Could you check a few things on this model? Use its own coordinates, in mm. Face numbers are marked on the shaded views. Round coordinates to 2 decimals unless told otherwise and drop trailing zeros. Order: outer loops, then holes, each group sorted by start corner. A loop starts at its lowest first (then second) coordinate and runs counter-clockwise, first axis right, second up. Notation, with made-up numbers: M 41,-35.5 L 53,-35.5 A25 ccw 53,-2.5 Z; hole C 24,6.25 d10. An arc over 180 degrees is marked long. Write each question's results on one line, items separated by ' | '. Start each with the question number.
1. Please list where these lines run through material, in increasing order: L1, parallel to Y at x = -6, z = 0.2; L2, parallel to Y at x = -1, z = 2.4; L3, parallel to X at y = 0, z = 1.25.
2. Suppose I cut it at D-D on x = -4. Write out the boundary of the cut face in (y, z), and give its area (3 significant figures).
3. Suppose I cut it at C-C on x = 1. Write out the boundary of the cut face in (y, z).
4. Suppose I cut it at B-B on z = 0.65. Write out the boundary of the cut face in (x, y).
5. Suppose I cut it at A-A on y = 0.25. Write out the boundary of the cut face in (x, z).
6. I'm going to push a flat-ended pin straight in: pin 1 (4.5 mm diameter, centred on x = 1.3, y = 1.38, fed in from -Z). Where does the tip first touch, or does it pass through?
7. We'd pull the mould along Y, two halves only. Please class the marked faces 1 and 2: released by +Y, released by -Y, zero draft, split by the parting line, or undercut.
from build123d import *

# Parameters (mm, degrees)
F1_DEPTH = 3


with BuildPart() as f1:
    # F0 (on Top) → F1 (new body)
    with BuildSketch(Plane.XY):
        with BuildLine():
            ThreePointArc((3.175484, -1.698676), (-2.295284, 1.377072), (3.175484, 4.452821))
            Line((3.175484, 4.452821), (3.175484, 6.121567))
            ThreePointArc((3.175484, 6.121567), (-1.151965, 5.846381), (-3.703487, 2.340347))
            ThreePointArc((-3.703487, 2.340347), (-4.972885, 3.651534), (-6.795181, 3.750636))
            Line((-6.795181, 3.750636), (-6.752376, 2.047452))
            ThreePointArc((-6.752376, 2.047452), (-5.010425, 1.376998), (-6.752376, 0.706545))
            Line((-6.752376, 0.706545), (-6.752376, -1.010366))
            ThreePointArc((-6.752376, -1.010366), (-4.952455, -0.888107), (-3.703468, 0.413697))
            ThreePointArc((-3.703468, 0.413697), (-1.15192, -3.092261), (3.175484, -3.367422))
            Line((3.175484, -3.367422), (3.175484, -1.698676))
        make_face()
    extrude(amount=F1_DEPTH)


solid = f1.part
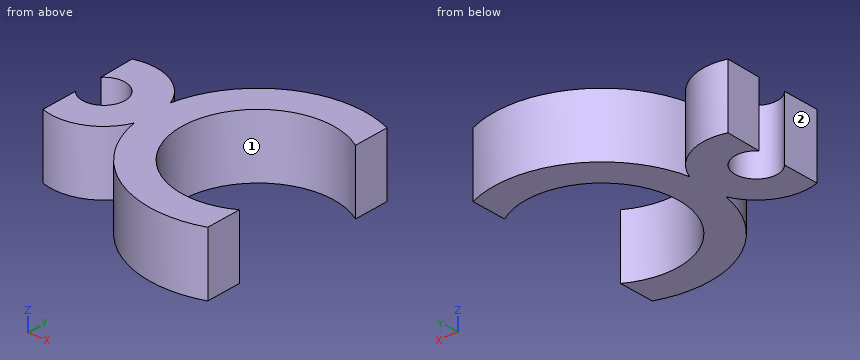
Filled sheet:
1) L1: y = -1.12 to 0.38, 2.38 to 3.88 | L2: y = -3.17 to -1.39, 4.14 to 5.93 | L3: x = -6.75 to -3.92, -3.61 to -2.02
2) outline: M -0.11,0 L 2.86,0 L 2.86,3 L -0.11,3 Z | area: 8.92 mm^2
3) outline: M -3.71,0 L -2.21,0 L -2.21,3 L -3.71,3 Z; M 4.96,0 L 6.47,0 L 6.47,3 L 4.96,3 Z
4) outline: M -6.8,3.75 L -6.75,2.05 A1 cw long -6.75,0.71 L -6.75,-1.01 A2.5 ccw -3.7,0.41 A5.1 ccw 3.18,-3.37 L 3.18,-1.7 A3.6 cw long 3.18,4.45 L 3.18,6.12 A5.1 ccw -3.7,2.34 A2.5 ccw Z
5) outline: M -6.75,0 L -3.78,0 L -3.78,3 L -6.75,3 Z; M -3.67,0 L -2.11,0 L -2.11,3 L -3.67,3 Z
6) pin 1: passes through
7) face 1: undercut | face 2: zero draft
